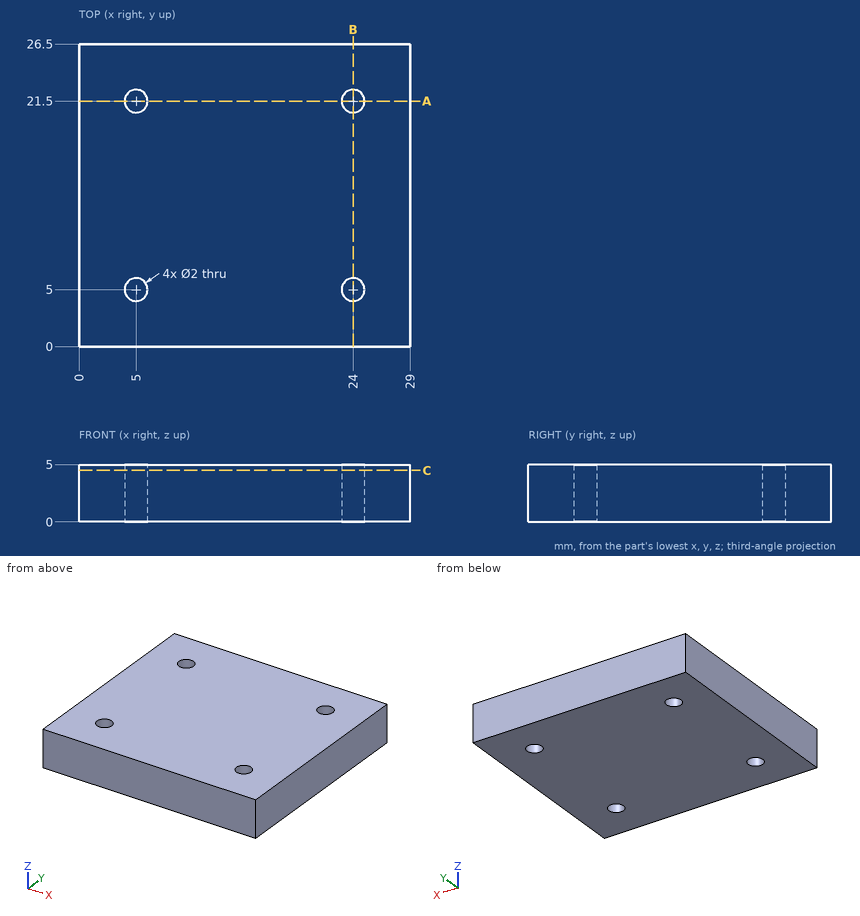
Input: dimensioned drawing with shaded views. Units: mm. Origin: part minimum x, y, z. Give positions to 0.01 mm unless a question says otherwise; leave off trailing zeros. Write each loop counter-clockwise with the first axis right and the second up, starting at its lowest first coordinate (ties: lowest second). Pieces come first, ordered by that corner, then holes. Notation, with made-up numbers: (0.5, 83.25) -> (12.5, 83.25) arc R20 cw to (12.5, 101.25) -> close; hole circle Ø4 at (25.5, 14.5). An arc over 180 degrees is marked (long way). Return JSON: item names as keys, results as strings. Group by question number.
1. Section B-B, the plane x = 24. Output: boundary loops of the cut face in (y, z), then the cut area to 4 significant figures.
2. Section C-C, the plane z = 4.5. Output: boundary loops of the cut face in (x, y).
3. Material intervals for line 1 (X direction, y = 21.5, z = 2.65); line 2 (Y direction, x = 5, z = 1.5), sorted ascending. Write a range as from..to.
4. Section A-A, the plane y = 21.5. Output: boundary loops of the cut face in (x, z).
Determined:
{
 "1": {"outline": "(0, 0) -> (4, 0) -> (4, 5) -> (0, 5) -> close; (6, 0) -> (20.5, 0) -> (20.5, 5) -> (6, 5) -> close; (22.5, 0) -> (26.5, 0) -> (26.5, 5) -> (22.5, 5) -> close", "area": "112.5 mm2"},
 "2": {"outline": "(0, 0) -> (29, 0) -> (29, 26.5) -> (0, 26.5) -> close; hole circle Ø2 at (5, 5); hole circle Ø2 at (5, 21.5); hole circle Ø2 at (24, 5); hole circle Ø2 at (24, 21.5)"},
 "3": {"line 1": "x = 0..4, 6..23, 25..29", "line 2": "y = 0..4, 6..20.5, 22.5..26.5"},
 "4": {"outline": "(0, 0) -> (4, 0) -> (4, 5) -> (0, 5) -> close; (6, 0) -> (23, 0) -> (23, 5) -> (6, 5) -> close; (25, 0) -> (29, 0) -> (29, 5) -> (25, 5) -> close"}
}
